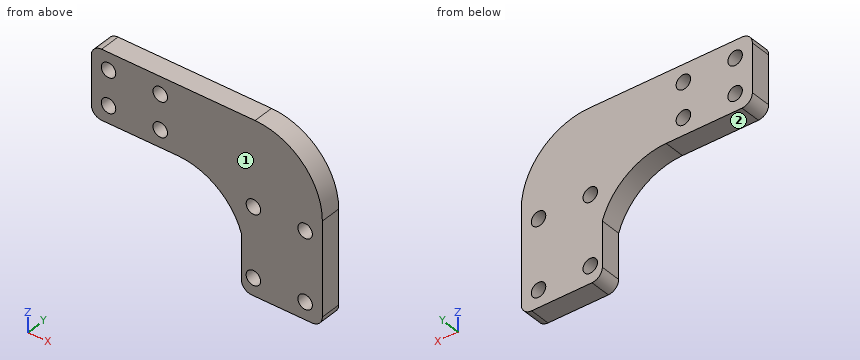
from build123d import *

# Parameters (mm, degrees)
SKETCH_1_R      = 2.1
EXTRUDE_1_DEPTH = 6
FILLET_1_R      = 3


with BuildPart() as part:
    # 草图1 → 凸台-拉伸1 (new body)
    with BuildSketch(Plane(origin=(0, 0, 0), x_dir=(1, 0, 0), z_dir=(0, 1, 0))):
        with BuildLine():
            Line((-11, 15), (12.5, 15))
            Line((12.5, 15), (12.5, -15))
            ThreePointArc((12.5, -15), (6.788582233, -28.788582233), (-7, -34.5))
            Line((-7, -34.5), (-54.5, -34.5))
            Line((-54.5, -34.5), (-54.5, -14.5))
            Line((-54.5, -14.5), (-29.5, -14.5))
            ThreePointArc((-29.5, -14.5), (-18.049017509, -10.766161191), (-11, -1))
            Line((-11, -1), (-11, 15))
        make_face()
        with Locations((-49.5, -19.5)):
            Circle(SKETCH_1_R, mode=Mode.SUBTRACT)
        with Locations((-7.5, -10)):
            Circle(SKETCH_1_R, mode=Mode.SUBTRACT)
        with Locations((-34.5, -19.5)):
            Circle(SKETCH_1_R, mode=Mode.SUBTRACT)
        with Locations((-34.5, -29.5)):
            Circle(SKETCH_1_R, mode=Mode.SUBTRACT)
        with Locations((-49.5, -29.5)):
            Circle(SKETCH_1_R, mode=Mode.SUBTRACT)
        with Locations((7.5, -10)):
            Circle(SKETCH_1_R, mode=Mode.SUBTRACT)
        with Locations((7.5, 10)):
            Circle(SKETCH_1_R, mode=Mode.SUBTRACT)
        with Locations((-7.5, 10)):
            Circle(SKETCH_1_R, mode=Mode.SUBTRACT)
    extrude(amount=EXTRUDE_1_DEPTH)

    # 圆角1
    fillet_1_edges = [part.edges().sort_by_distance(p)[0] for p in [
        (-11, 3, -15),
        (12.5, 3, -15),
        (-54.5, 3, 34.5),
        (-54.5, 3, 14.5),
    ]]
    fillet(fillet_1_edges, radius=FILLET_1_R)


solid = part.part
Here's how the part is built. I have some questions about the finished solid (model axes, mm). Face numbers are marked on the shaded views. A direction names the side the tool comes from. Coordinates: 2 decimals unless noted, no trailing zeros. Order: outer loops, then holes, each group sorted by start corner. A loop starts at its lowest first (then second) coordinate and runs counter-clockwise, first axis right, second up.
Item 1: If we section it at D-D on z = -2.5: List the corners of the cut face in (x, y) for me, plus the area to 3 significant figures.
Result sheet:
outline: (-11, 0) - (12.5, 0) - (12.5, 6) - (-11, 6) - close
area: 141 mm2
Item 2: I need wall thicknesses on line 1 (Z direction, x = -7.5, y = 3.55); line 2 (Z direction, x = -49.5, y = 3.65); line 3 (X direction, y = 3.85, z = 10). Which ranges of each line are inside material? Lowest first, please.
Result sheet:
line 1: z = -15 to -12.1, -7.9 to 7.9, 12.1 to 34.5
line 2: z = 14.5 to 17.4, 21.6 to 27.4, 31.6 to 34.5
line 3: x = -17.07 to -9.6, -5.4 to 5.4, 9.6 to 12.5
Item 3: If we section it at B-B on z = -10: List the corners of the cut face in (x, y) for me, plus the area to 3 significant figures.
Result sheet:
outline: (-11, 0) - (-9.6, 0) - (-9.6, 6) - (-11, 6) - close; (-5.4, 0) - (5.4, 0) - (5.4, 6) - (-5.4, 6) - close; (9.6, 0) - (12.5, 0) - (12.5, 6) - (9.6, 6) - close
area: 90.6 mm2
Item 4: If we section it at C-C on y = 3.75: State how many separate pieces and enclosed holes the cut face has, plus the area to 3 significant figures.
Result sheet:
separate pieces: 1
enclosed holes: 8
area: 1,900 mm2
Item 5: For P1, Ø1.8, axis at y = 3.5, z = -7.5, coming from the -X side; P2, Ø3, axis at x = -36, y = 4, coming from the -Z side, each with a flat end and sliding along its axis, tell me the tip position at first contact or that it passes through.
Result sheet:
P1: stops at x = -11
P2: stops at z = 14.5
Item 6: If we section it at A-A on x = -49.5: List the corners of the cut face in (y, z) for me.
Result sheet:
outline: (0, 14.5) - (6, 14.5) - (6, 17.4) - (0, 17.4) - close; (0, 21.6) - (6, 21.6) - (6, 27.4) - (0, 27.4) - close; (0, 31.6) - (6, 31.6) - (6, 34.5) - (0, 34.5) - close
Item 7: For the marked faces 1 and 2, which set-ups out of +Z, -Z, +X, -X, +Y, -Y let a thin tool reach every point of the face, with its end or its side?
Result sheet:
face 1: +Z, -Z, +X, -X, -Y
face 2: -Z, -X, +Y, -Y
